Part model, mm, in its own coordinate system. A direction names the side the tool comes from. Round coordinates to 2 decimals unless told otherwise and drop trailing zeros. Loops run counter-clockwise (first coordinate to the right, second up) from the corner with the lowest first, then second, coordinate; pieces in that order, holes last. Notation, with made-up numbers: M -40,41.25 L -12,41.25 A16 cw -12,62.25 Z; hole C 5,-10.75 d8. An arc over 180 degrees is marked long. Answer as CSV lines item,"result". Start each with the question number.
Item 1: Which spindle directions (+Z, -Z, +X, -X, +Y, -Y) get a long thin tool onto all of the face, cutting with end or side? Do faces 4 (the flat face through (9, 0, -13)), 5 (the cylindrical face through (74.774, 20.721, 1.014)), 6 (the flat face through (-40, 3.175, -10)), 7 (the flat face through (39, -3.175, -10)). Say none if no direction does.
Item 2: Band-saw the part on B-B (x = 48). Give the cut face in (y, z) (3 decimals).
Item 3: Band-saw the part on D-D (x = 0). Give the cut face in (y, z) (3 decimals).
Item 4: Wall check: line 1 (Y direction, x = 48, z = 0.1) (3 decimals); line 2 (X direction, y = -12.7, z = 0.1); line 3 (X direction, y = -12.7, z = 0.25). Give the ranges that are in metal, low to high.
Item 5: Band-saw the part on A-A (y = -12.7). Give the cut face in (x, z).
Item 6: Band-saw the part on C-C (z = -5.5). Give the cut face in (x, y) (3 decimals), and give its area (3 significant figures).
Item 7: Drop flat-ended pins along their axis: pin 1 Ø5.5 at (x, z) = (56.5, -11.5) entering from -Y (3 decimals); pin 2 Ø2 at (x, y) = (-48.5, -16.5) entering from -Z. Give the stop position or say it passes through.
Item 8: Mould opens along X. For faces 1 (the cylindrical face through (74.774, -20.721, 1.014)), 2 (the cylindrical face through (0.2, -0.1, -0.4)), 3 (the flat face through (-76.2, 0, -4)) say: pulls with the +X half, pulls with the -X half, needs draft (parallel to the pull), parting line crosses it, or undercut.
```python
from build123d import *

# Parameters (mm, degrees)
F0_W         = 152.4
F0_H         = 44.45
F1_DEPTH     = 2
F2_W         = 152.4
F2_H         = 6.35
F3_DEPTH     = 18.796
F4_R         = 1.75
F5_DEPTH     = 25
F7_DEPTH     = 25.401
F8_SIZE      = 1.8
F9_T4_DEPTH  = 152.4
F9_S5_R      = 9
F9_T6_DEPTH  = 78
F9_T10_DEPTH = 152.4
F9_S11_R     = 9
F9_T12_DEPTH = 78
F10_R        = 2
F11_R        = 5


# Not quite as in the source:
# - a fillet or chamfer that OpenCascade refuses, or shapes differently, is made with other operations: its cross-section is extruded or revolved along the edge and cut away or added
# - a feature names something its author has since deleted; it is built from what else it names


with BuildPart() as f1:
    # F0 (on Top) → F1 (new body)
    with BuildSketch(Plane.XY):
        Rectangle(F0_W, F0_H)
    extrude(amount=F1_DEPTH)

    # F2 (on face) → F3 (join)
    with BuildSketch(Plane(origin=(0, 0, 0), x_dir=(1, 0, 0), z_dir=(0, 0, -1))):
        Rectangle(F2_W, F2_H)
    extrude(amount=F3_DEPTH)

    # F4 (on face) → F5 (cut)
    with BuildSketch(Plane(origin=(0, 0, 0), x_dir=(1, 0, 0), z_dir=(0, 0, -1))):
        with Locations((48, -12.7)):
            Circle(F4_R)
        with Locations((-48, -12.7)):
            Circle(F4_R)
        with Locations((-48, 12.7)):
            Circle(F4_R)
        with Locations((48, 12.7)):
            Circle(F4_R)
    extrude(amount=-F5_DEPTH, mode=Mode.SUBTRACT)

    # F6 (on face) → F7 (cut, through all)
    with BuildSketch(Plane(origin=(0, 3.175, 0), x_dir=(-1, 0, 0), z_dir=(0, 1, 0))):
        with BuildLine():
            ThreePointArc((-9, -9.398), (0, -18.398), (9, -9.398))
            ThreePointArc((9, -9.398), (0, -0.398), (-9, -9.398))
        make_face()
        with BuildLine():
            Line((9, -18.796), (9, -9.398))
            ThreePointArc((9, -9.398), (0, -18.398), (-9, -9.398))
            Line((-9, -9.398), (-9, -18.796))
            Line((-9, -18.796), (9, -18.796))
        make_face()
    extrude(amount=-F7_DEPTH, mode=Mode.SUBTRACT)

    # F8
    f8_edges = [f1.edges().sort_by_distance(p)[0] for p in [
        (46.25, -12.7, 2),
        (-49.75, -12.7, 2),
        (-49.75, 12.7, 2),
        (46.25, 12.7, 2),
    ]]
    chamfer(f8_edges, length=F8_SIZE)

    # F9: chamfer of 1 on 2 edges, made by hand


with BuildPart() as f9_tool2:
    # F9_s3 → F9_t4 (new body)
    with BuildSketch(Plane.YZ.offset(-76.2)):
        Polygon((3.175, -1), (4.175, 0), (3.175, 0), align=None)
    extrude(amount=F9_T4_DEPTH)

    # F9_s5 → F9_t6 (cut, symmetric)
    with BuildSketch(Plane.XZ.offset(-3.7)):
        with Locations((0, -9.398)):
            Circle(F9_S5_R)
    extrude(amount=F9_T6_DEPTH, both=True, mode=Mode.SUBTRACT)


with BuildPart() as f1_1:
    add(f1.part)

    # F9_t1: union F9_tool2
    add(f9_tool2.part)


with BuildPart() as f9_tool8:
    # F9_s9 → F9_t10 (new body)
    with BuildSketch(Plane.YZ.offset(76.2)):
        Polygon((-4.175, 0), (-3.175, -1), (-3.175, 0), align=None)
    extrude(amount=-F9_T10_DEPTH)

    # F9_s11 → F9_t12 (cut, symmetric)
    with BuildSketch(Plane.XZ.offset(3.7)):
        with Locations((0, -9.398)):
            Circle(F9_S11_R)
    extrude(amount=F9_T12_DEPTH, both=True, mode=Mode.SUBTRACT)


with BuildPart() as f1_2:
    add(f1_1.part)

    # F9_t7: union F9_tool8
    add(f9_tool8.part)

    # F10
    f10_edges = [f1_2.edges().sort_by_distance(p)[0] for p in [
        (9, 0, -18.796),
        (-9, 0, -18.796),
    ]]
    fillet(f10_edges, radius=F10_R)

    # F11
    f11_edges = [f1_2.edges().sort_by_distance(p)[0] for p in [
        (76.2, 0, -18.796),
        (76.2, -22.225, 1),
        (76.2, 22.225, 1),
    ]]
    fillet(f11_edges, radius=F11_R)


solid = f1_2.part
```
Answer block:
1,face 4,"-Z, +Y, -Y"
1,face 5,"+Z, -Z, +X, +Y"
1,face 6,"-Z, +X, -X, +Y"
1,face 7,"-Z, +X, -X, -Y"
2,outline,"M -22.225,0 L -14.45,0 L -14.45,0.2 L -16.25,2 L -22.225,2 Z; M -10.95,0 L -4.175,0 L -3.175,-1 L -3.175,-18.796 L 3.175,-18.796 L 3.175,-1 L 4.175,0 L 10.95,0 L 10.95,0.2 L 9.15,2 L -9.15,2 L -10.95,0.2 Z; M 14.45,0 L 22.225,0 L 22.225,2 L 16.25,2 L 14.45,0.2 Z"
3,outline,"M -22.225,0 L -4.175,0 L -3.777,-0.398 L 3.777,-0.398 L 4.175,0 L 22.225,0 L 22.225,2 L -22.225,2 Z"
4,line 1,"y = -22.225 to -14.45, -10.95 to 10.95, 14.45 to 22.225"
4,line 2,"x = -76.2 to -49.75, -46.25 to 46.25, 49.75 to 76.2"
4,line 3,"x = -76.2 to -49.8, -46.2 to 46.2, 49.8 to 76.2"
5,outline,"M -76.2,0 L -49.75,0 L -49.75,0.2 L -51.55,2 L -76.2,2 Z; M -46.25,0 L 46.25,0 L 46.25,0.2 L 44.45,2 L -44.45,2 L -46.25,0.2 Z; M 49.75,0 L 76.2,0 L 76.2,2 L 51.55,2 L 49.75,0.2 Z"
6,outline,"M -76.2,-3.175 L -8.112,-3.175 L -8.112,3.175 L -76.2,3.175 Z; M 8.112,-3.175 L 76.2,-3.175 L 76.2,3.175 L 8.112,3.175 Z"
6,area,"865 mm^2"
7,pin 1,"stops at y = -3.175"
7,pin 2,"stops at z = 0"
8,face 1,"pulls with the +X half"
8,face 2,"undercut"
8,face 3,"pulls with the -X half"
